from build123d import *

# Parameters (mm, degrees)
F0_W      = 15.875
F0_H      = 25.4
F0_H_2    = 1451.4265329467
F0_H_3    = 25.4000000258
F0_W_2    = 31.75
F0_H_4    = 76.2
F0_H_5    = 11.7933667633
F0_H_6    = 11.7933667375
F1_DEPTH  = 508
F2_START  = -76.2
F1_FACE_W = 31.75
F1_FACE_H = 1676.4
F2_DEPTH  = 355.6
F3_DEPTH  = 508
F4_DEPTH  = 508
F5_START  = 31.75
F5_DEPTH  = 444.5


with BuildPart() as f1:
    # F0 (on Front) → F1 (new body)
    with BuildSketch(Plane.XZ):
        with Locations((357.1875, 1448.0473103974)):
            Rectangle(F0_W, F0_H)
        Polygon((381, 1423.553943634), (381, 1497.9406771607), (349.25, 1497.9406771607), (349.25, 1460.7473103974), (365.125, 1460.7473103974), (365.125, 1435.3473103974), (365.125, 1423.553943634), align=None)
        with Locations((373.0625, 697.8406771607)):
            Rectangle(F0_W, F0_H_2)
        with Locations((357.1875, 697.8406771607)):
            Rectangle(F0_W, F0_H_2)
        Polygon((381, -102.2593228393), (381, -27.8725893126), (365.125, -27.8725893126), (365.125, -39.6659560502), (365.125, -65.065956076), (349.25, -65.065956076), (349.25, -102.2593228393), align=None)
        with Locations((357.1875, -52.3659560631)):
            Rectangle(F0_W, F0_H_3)
        with Locations((365.125, -140.3593228393)):
            Rectangle(F0_W_2, F0_H_4)
        with Locations((357.1875, 1429.4506270157)):
            Rectangle(F0_W, F0_H_5)
        with Locations((357.1875, -33.7692726814)):
            Rectangle(F0_W, F0_H_6)
    extrude(amount=F1_DEPTH)


with BuildPart() as f1b:
    # F0 (on Front) → F1, piece 2 (new body)
    with BuildSketch(Plane.XZ):
        with Locations((-365.125, -140.3593228393)):
            Rectangle(F0_W_2, F0_H_4)
        Polygon((-365.125, -27.8725893126), (-381, -27.8725893126), (-381, -102.2593228393), (-349.25, -102.2593228393), (-349.25, -65.065956076), (-365.125, -65.065956076), (-365.125, -39.6659560502), align=None)
        with Locations((-357.1875, -52.3659560631)):
            Rectangle(F0_W, F0_H_3)
        with Locations((-357.1875, 697.8406771607)):
            Rectangle(F0_W, F0_H_2)
        with Locations((-373.0625, 697.8406771607)):
            Rectangle(F0_W, F0_H_2)
        with Locations((-357.1875, 1448.0473103974)):
            Rectangle(F0_W, F0_H)
        Polygon((-349.25, 1460.7473103974), (-349.25, 1497.9406771607), (-381, 1497.9406771607), (-381, 1423.553943634), (-365.125, 1423.553943634), (-365.125, 1435.3473103974), (-365.125, 1460.7473103974), align=None)
        with Locations((-357.1875, 1429.4506270157)):
            Rectangle(F0_W, F0_H_5)
        with Locations((-357.1875, -33.7692726814)):
            Rectangle(F0_W, F0_H_6)
    extrude(amount=F1_DEPTH)


with BuildPart() as f2_tool:
    # F1_face (on face) → F2 (new body)
    with BuildSketch(Plane(origin=(365.125, 0, 659.7406771607), x_dir=(1, 0, 0), z_dir=(0, 1, 0)).offset(F2_START)):
        Rectangle(F1_FACE_W, F1_FACE_H)
        with Locations((-730.25, 0)):
            Rectangle(F1_FACE_W, F1_FACE_H)
    extrude(amount=-F2_DEPTH)


with BuildPart() as f1_1:
    add(f1.part)

    # F2: cut by f2_tool
    add(f2_tool.part, mode=Mode.SUBTRACT)



with BuildPart() as f1b_1:
    add(f1b.part)

    # F2: cut by f2_tool
    add(f2_tool.part, mode=Mode.SUBTRACT)


with BuildPart() as f3:
    # F0 (on Front) → F3 (new body, through all)
    with BuildSketch(Plane.XZ):
        Polygon((381, 1423.553943634), (381, 1497.9406771607), (349.25, 1497.9406771607), (349.25, 1460.7473103974), (365.125, 1460.7473103974), (365.125, 1435.3473103974), (365.125, 1423.553943634), align=None)
        with Locations((357.1875, 1429.4506270157)):
            Rectangle(F0_W, F0_H_5)
        with Locations((357.1875, 1448.0473103974)):
            Rectangle(F0_W, F0_H)
    extrude(amount=F3_DEPTH)


with BuildPart() as f3b:
    # F0 (on Front) → F3, piece 2 (new body, through all)
    with BuildSketch(Plane.XZ):
        Polygon((-349.25, 1460.7473103974), (-349.25, 1497.9406771607), (-381, 1497.9406771607), (-381, 1423.553943634), (-365.125, 1423.553943634), (-365.125, 1435.3473103974), (-365.125, 1460.7473103974), align=None)
        with Locations((-357.1875, 1448.0473103974)):
            Rectangle(F0_W, F0_H)
        with Locations((-357.1875, 1429.4506270157)):
            Rectangle(F0_W, F0_H_5)
    extrude(amount=F3_DEPTH)


with BuildPart() as f3c:
    # F0 (on Front) → F3, piece 3 (new body, through all)
    with BuildSketch(Plane.XZ):
        with Locations((357.1875, -52.3659560631)):
            Rectangle(F0_W, F0_H_3)
        Polygon((381, -102.2593228393), (381, -27.8725893126), (365.125, -27.8725893126), (365.125, -39.6659560502), (365.125, -65.065956076), (349.25, -65.065956076), (349.25, -102.2593228393), align=None)
        with Locations((357.1875, -33.7692726814)):
            Rectangle(F0_W, F0_H_6)
    extrude(amount=F3_DEPTH)


with BuildPart() as f3d:
    # F0 (on Front) → F3, piece 4 (new body, through all)
    with BuildSketch(Plane.XZ):
        with Locations((-357.1875, -52.3659560631)):
            Rectangle(F0_W, F0_H_3)
        Polygon((-365.125, -27.8725893126), (-381, -27.8725893126), (-381, -102.2593228393), (-349.25, -102.2593228393), (-349.25, -65.065956076), (-365.125, -65.065956076), (-365.125, -39.6659560502), align=None)
        with Locations((-357.1875, -33.7692726814)):
            Rectangle(F0_W, F0_H_6)
    extrude(amount=F3_DEPTH)


with BuildPart() as f1_2:
    add(f1_1.part)

    add(f1b_1.part)  # F4 merges F1b

    add(f3.part)  # F4 merges F3

    add(f3b.part)  # F4 merges F3b

    add(f3c.part)  # F4 merges F3c

    add(f3d.part)  # F4 merges F3d
    # F0 (on Front) → F4 (join)
    with BuildSketch(Plane.XZ):
        Polygon((349.25, 1460.7473103974), (349.25, 1497.9406771607), (-349.25, 1497.9406771607), (-349.25, 1460.7473103974), (0, 1460.7473103974), align=None)
        Polygon((349.25, 1423.553943634), (349.25, 1435.3473103974), (0, 1435.3473103974), (-349.25, 1435.3473103974), (-349.25, 1423.553943634), align=None)
        Polygon((349.25, -39.6659560502), (349.25, -27.8725893126), (-349.25, -27.8725893126), (-349.25, -39.6659560502), (0, -39.6659560502), align=None)
        Polygon((-349.25, -102.2593228393), (349.25, -102.2593228393), (349.25, -65.065956076), (0, -65.065956076), (-349.25, -65.065956076), align=None)
        Polygon((0, -65.065956076), (349.25, -65.065956076), (349.25, -39.6659560502), (0, -39.6659560502), (-349.25, -39.6659560502), (-349.25, -65.065956076), align=None)
        Polygon((349.25, 1435.3473103974), (349.25, 1460.7473103974), (0, 1460.7473103974), (-349.25, 1460.7473103974), (-349.25, 1435.3473103974), (0, 1435.3473103974), align=None)
    extrude(amount=F4_DEPTH)

    # F0 (on Front) → F5 (cut)
    with BuildSketch(Plane.XZ.offset(F5_START)):
        Polygon((349.25, 1423.553943634), (349.25, 1435.3473103974), (0, 1435.3473103974), (-349.25, 1435.3473103974), (-349.25, 1423.553943634), align=None)
        Polygon((349.25, 1460.7473103974), (349.25, 1497.9406771607), (-349.25, 1497.9406771607), (-349.25, 1460.7473103974), (0, 1460.7473103974), align=None)
        Polygon((349.25, -39.6659560502), (349.25, -27.8725893126), (-349.25, -27.8725893126), (-349.25, -39.6659560502), (0, -39.6659560502), align=None)
        Polygon((-349.25, -102.2593228393), (349.25, -102.2593228393), (349.25, -65.065956076), (0, -65.065956076), (-349.25, -65.065956076), align=None)
        Polygon((349.25, 1435.3473103974), (349.25, 1460.7473103974), (0, 1460.7473103974), (-349.25, 1460.7473103974), (-349.25, 1435.3473103974), (0, 1435.3473103974), align=None)
        Polygon((0, -65.065956076), (349.25, -65.065956076), (349.25, -39.6659560502), (0, -39.6659560502), (-349.25, -39.6659560502), (-349.25, -65.065956076), align=None)
    extrude(amount=F5_DEPTH, mode=Mode.SUBTRACT)


solid = f1_2.part
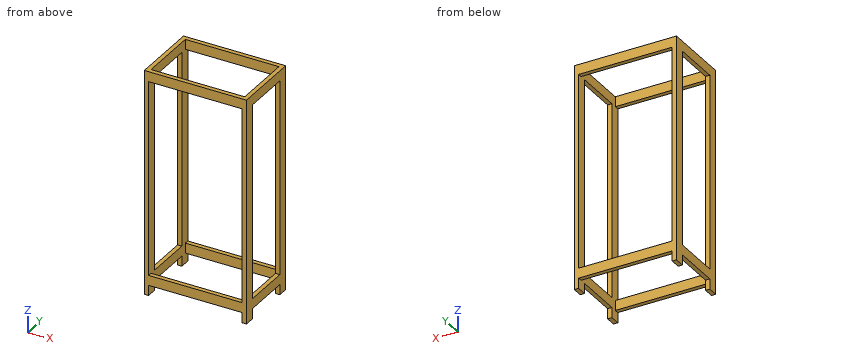
Build history of the part. All positions in model axes, mm. Give positions to 0.01 mm unless a question says otherwise; leave off trailing zeros. Write each loop counter-clockwise with the first axis right and the second up, starting at its lowest first coordinate (ties: lowest second). Pieces come first, ordered by that corner, then holes. Notation, with made-up numbers: (-26.5, 47.5) - (29.5, 47.5) arc R17 cw to (29.5, 71.5) - close; hole circle Ø8 at (16.25, 68). An arc over 180 degrees is marked (long way). Use one line per item in the form item = value. Start each with the question number.
1. Band-saw the part on B-B on y = -105. Write the cut outline in (x, z).
2. Band-saw the part on A-A on x = -2.5. Write the cut outline in (y, z).
3. Probe line 1 (X direction, y = -62.5, z = 168.5); line 2 (Z direction, x = 11.5, y = -21.5). List the from-to ranges inside material, lowest first. Write a range as [from, to].
4. Drop a flat-ended pin along its axis: pin 1 Ø16 at (x, z) = (-369.5, -142.5) entering from +Y. Give the stop position or say it passes through.
Conclusion:
q1.outline = (-381, -102.26) - (-349.25, -102.26) - (-349.25, -27.87) - (-381, -27.87) - close; (-381, 1423.55) - (-349.25, 1423.55) - (-349.25, 1497.94) - (-381, 1497.94) - close; (349.25, -102.26) - (381, -102.26) - (381, -27.87) - (349.25, -27.87) - close; (349.25, 1423.55) - (381, 1423.55) - (381, 1497.94) - (349.25, 1497.94) - close
q2.outline = (-508, -102.26) - (-476.25, -102.26) - (-476.25, -27.87) - (-508, -27.87) - close; (-508, 1423.55) - (-476.25, 1423.55) - (-476.25, 1497.94) - (-508, 1497.94) - close; (-31.75, -102.26) - (0, -102.26) - (0, -27.87) - (-31.75, -27.87) - close; (-31.75, 1423.55) - (0, 1423.55) - (0, 1497.94) - (-31.75, 1497.94) - close
q3.line_1 = [-381, -349.25], [349.25, 381]
q3.line_2 = [-102.26, -27.87], [1423.55, 1497.94]
q4.pin_1 = 0
